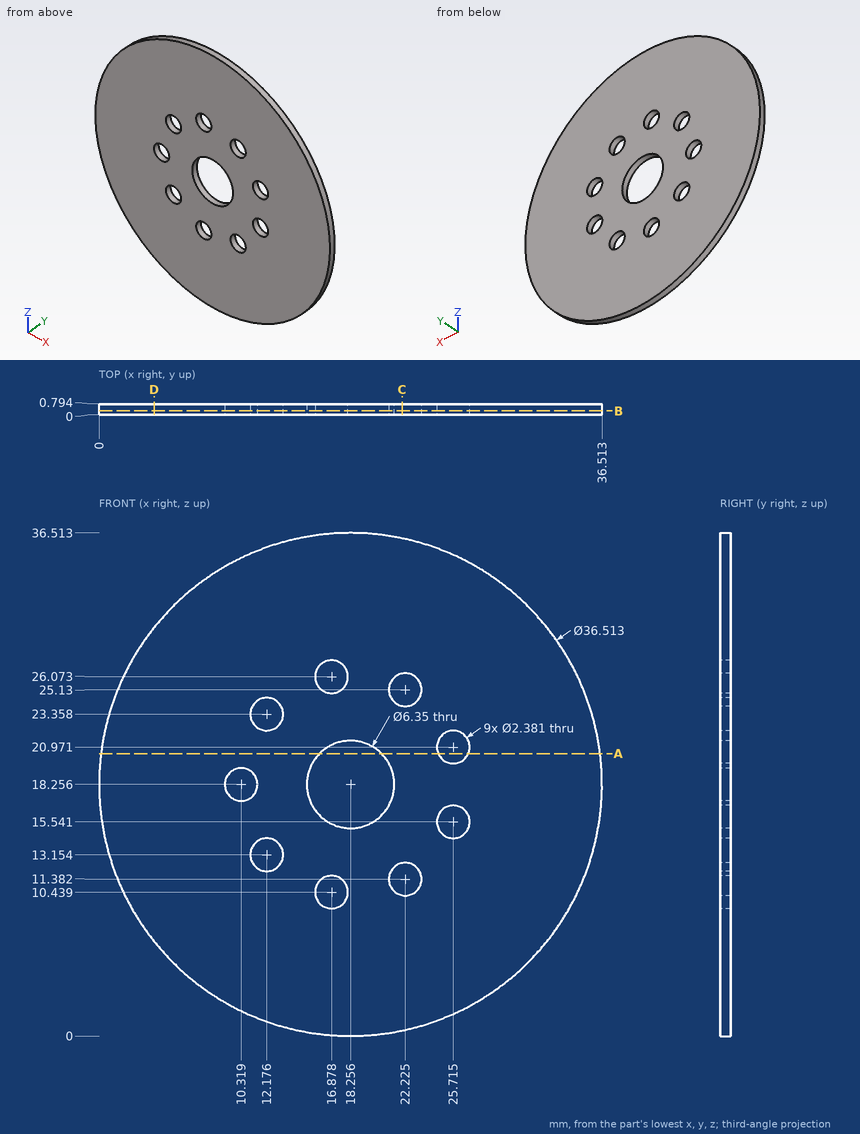
Geometry: see drawing. Coordinates: mm, zero at the bounding-box minimum. Round coordinates to 2 decimals unless told otherwise and drop trailing zeros. Loops run counter-clockwise (first coordinate to the right, second up) from the corner with the lowest first, then second, coordinate; pieces in that order, holes last. Notation, with made-up numbers: M 75.25,-9 L 107.25,-9 A17 ccw 107.25,-3 Z; hole C 56,-26 d2. An arc over 180 degrees is marked long. Use a Markdown table: item, result. Add a question column.
1. Section query A-A on z = 20.5. Return the cut outline in (x, y) (1 decimal).
2. Line query: line 1 (X direction, y = 0.4, z = 16) (1 decimal); line 2 (Z direction, x = 21.5, y = 0.4) (1 decimal); line 3 (X direction, y = 0.7, z = 25.5) (1 decimal). Output: solid intervals per line, ascending.
3. Contact query for a flat-ended pin moving along its axis: P1, Ø4, axis at x = 16.88, z = 26.07, coming from the -Y side. Output: stop coordinate, or through.
4. Section query D-D on x = 4. Return the cut outline in (y, z).
5. Section query C-C on x = 22. Return the cut outline in (y, z) (1 decimal).
6. Section query B-B on y = 0.3. Give the number of separate pieces and of enclosed holes in the cut face.
Reported:
| question | item | result |
|---|---|---|
| 1 | outline | M 0.1,0 L 16,0 L 16,0.8 L 0.1,0.8 Z; M 20.5,0 L 24.6,0 L 24.6,0.8 L 20.5,0.8 Z; M 26.8,0 L 36.4,0 L 36.4,0.8 L 26.8,0.8 Z |
| 2 | line 1 | x = 0.1 to 16, 20.5 to 24.6, 26.8 to 36.4 |
| 2 | line 2 | z = 0.3 to 10.4, 12.3 to 24.2, 26.1 to 36.2 |
| 2 | line 3 | x = 1.5 to 15.8, 17.9 to 21.1, 23.4 to 35 |
| 3 | P1 | stops at y = 0 |
| 4 | outline | M 0,6.85 L 0.79,6.85 L 0.79,29.66 L 0,29.66 Z |
| 5 | outline | M 0,0.4 L 0.8,0.4 L 0.8,10.2 L 0,10.2 Z; M 0,12.6 L 0.8,12.6 L 0.8,24 L 0,24 Z; M 0,26.3 L 0.8,26.3 L 0.8,36.1 L 0,36.1 Z |
| 6 | separate pieces | 1 |
| 6 | enclosed holes | 10 |
